from build123d import *

# Parameters (mm, degrees)
F1_DEPTH      = 1.5
F3_DEPTH      = 1.5
F4_W          = 1
F4_H          = 1
F4_W_2        = 0.5
F5_DEPTH      = 5
F5_DEPTH_BACK = 5
F6_COUNT      = 4
F6_ANGLE      = 270


with BuildPart() as f1:
    # F0 (on Top) → F1 (new body)
    with BuildSketch(Plane.XY):
        with BuildLine():
            ThreePointArc((16.8, 11), (15.1012193309, 15.1012193309), (11, 16.8))
            Line((11, 16.8), (-11, 16.8))
            ThreePointArc((-11, 16.8), (-15.1012193309, 15.1012193309), (-16.8, 11))
            Line((-16.8, 11), (-16.8, -11))
            ThreePointArc((-16.8, -11), (-15.1012193309, -15.1012193309), (-11, -16.8))
            Line((-11, -16.8), (11, -16.8))
            ThreePointArc((11, -16.8), (15.1012193309, -15.1012193309), (16.8, -11))
            Line((16.8, -11), (16.8, 11))
        make_face()
        with BuildLine():
            Line((-11, 15.3), (11, 15.3))
            ThreePointArc((11, 15.3), (14.0405591591, 14.0405591591), (15.3, 11))
            Line((15.3, 11), (15.3, -11))
            ThreePointArc((15.3, -11), (14.0405591591, -14.0405591591), (11, -15.3))
            Line((11, -15.3), (-11, -15.3))
            ThreePointArc((-11, -15.3), (-14.0405591591, -14.0405591591), (-15.3, -11))
            Line((-15.3, -11), (-15.3, 11))
            ThreePointArc((-15.3, 11), (-14.0405591591, 14.0405591591), (-11, 15.3))
        make_face(mode=Mode.SUBTRACT)
        with BuildLine():
            ThreePointArc((15.3, 11), (14.0405591591, 14.0405591591), (11, 15.3))
            Line((11, 15.3), (-11, 15.3))
            ThreePointArc((-11, 15.3), (-14.0405591591, 14.0405591591), (-15.3, 11))
            Line((-15.3, 11), (-15.3, -11))
            ThreePointArc((-15.3, -11), (-14.0405591591, -14.0405591591), (-11, -15.3))
            Line((-11, -15.3), (11, -15.3))
            ThreePointArc((11, -15.3), (14.0405591591, -14.0405591591), (15.3, -11))
            Line((15.3, -11), (15.3, 11))
        make_face()
        with BuildLine():
            Line((-11, 15), (11, 15))
            ThreePointArc((11, 15), (13.8284271247, 13.8284271247), (15, 11))
            Line((15, 11), (15, -11))
            ThreePointArc((15, -11), (13.8284271247, -13.8284271247), (11, -15))
            Line((11, -15), (-11, -15))
            ThreePointArc((-11, -15), (-13.8284271247, -13.8284271247), (-15, -11))
            Line((-15, -11), (-15, 11))
            ThreePointArc((-15, 11), (-13.8284271247, 13.8284271247), (-11, 15))
        make_face(mode=Mode.SUBTRACT)
        with BuildLine():
            ThreePointArc((15, 11), (13.8284271247, 13.8284271247), (11, 15))
            Line((11, 15), (-11, 15))
            ThreePointArc((-11, 15), (-13.8284271247, 13.8284271247), (-15, 11))
            Line((-15, 11), (-15, -11))
            ThreePointArc((-15, -11), (-13.8284271247, -13.8284271247), (-11, -15))
            Line((-11, -15), (11, -15))
            ThreePointArc((11, -15), (13.8284271247, -13.8284271247), (15, -11))
            Line((15, -11), (15, 11))
        make_face()
    extrude(amount=F1_DEPTH)

    # F2 (on face) → F3 (join)
    with BuildSketch(Plane.XY.offset(1.5)):
        with BuildLine():
            Line((16.8, -11), (16.8, 11))
            ThreePointArc((16.8, 11), (15.1012193309, 15.1012193309), (11, 16.8))
            Line((11, 16.8), (-11, 16.8))
            ThreePointArc((-11, 16.8), (-15.1012193309, 15.1012193309), (-16.8, 11))
            Line((-16.8, 11), (-16.8, -11))
            ThreePointArc((-16.8, -11), (-15.1012193309, -15.1012193309), (-11, -16.8))
            Line((-11, -16.8), (11, -16.8))
            ThreePointArc((11, -16.8), (15.1012193309, -15.1012193309), (16.8, -11))
        make_face()
        with BuildLine():
            Line((-11, 15.3), (11, 15.3))
            ThreePointArc((11, 15.3), (14.0405591591, 14.0405591591), (15.3, 11))
            Line((15.3, 11), (15.3, -11))
            ThreePointArc((15.3, -11), (14.0405591591, -14.0405591591), (11, -15.3))
            Line((11, -15.3), (-11, -15.3))
            ThreePointArc((-11, -15.3), (-14.0405591591, -14.0405591591), (-15.3, -11))
            Line((-15.3, -11), (-15.3, 11))
            ThreePointArc((-15.3, 11), (-14.0405591591, 14.0405591591), (-11, 15.3))
        make_face(mode=Mode.SUBTRACT)
    extrude(amount=F3_DEPTH)

    # F4 (on Front) → F5 (join, two sides)
    with BuildSketch(Plane.XZ) as f5_sk:
        with BuildLine():
            Line((-16.8, 10.5), (-16.8, 4))
            Line((-16.8, 4), (-15.8, 4))
            Line((-15.8, 4), (-15.8, 10.7488969095))
            ThreePointArc((-15.8, 10.7488969095), (-15.9830967627, 10.9326941499), (-16.2336477008, 11))
            Line((-16.2336477008, 11), (-16.3, 11))
            ThreePointArc((-16.3, 11), (-16.6535533906, 10.8535533906), (-16.8, 10.5))
        make_face()
        with Locations((-16.3, 3.5)):
            Rectangle(F4_W, F4_H)
        with Locations((-15.55, 3.5)):
            Rectangle(F4_W_2, F4_H)
        with BuildLine():
            Line((-15.8, 10.7488969095), (-15.8, 4))
            Line((-15.8, 4), (-15.3, 4))
            Line((-15.3, 4), (-15.3, 7.5))
            Line((-15.3, 7.5), (-15.738672954, 10.5707106781))
            ThreePointArc((-15.738672954, 10.5707106781), (-15.7608660432, 10.6627190959), (-15.8, 10.7488969095))
        make_face()
        with BuildLine():
            Line((-15.3, 7.5), (-15.3, 4))
            Line((-15.3, 4), (-14.848307792, 4))
            ThreePointArc((-14.848307792, 4), (-14.8342154179, 4.154457802), (-14.8441767052, 4.3092369361))
            Line((-14.8441767052, 4.3092369361), (-15.3, 7.5))
        make_face()
        with BuildLine():
            Line((-15.3, 4), (-15.3, 3))
            Line((-15.3, 3), (-14.9396990078, 3.7206019844))
            ThreePointArc((-14.9396990078, 3.7206019844), (-14.8836806771, 3.8569244249), (-14.848307792, 4))
            Line((-14.848307792, 4), (-15.3, 4))
        make_face()
    extrude(amount=F5_DEPTH)
    extrude(f5_sk.sketch, amount=-F5_DEPTH_BACK)

    # F6: F1 ×4 about axis
    f6_axis = Axis((0, 0, 16.5911819786), (0, 0, 1))


with BuildPart() as f1_1:
    add(f1.part)
    for i in range(1, F6_COUNT):
        add(f1.part.rotate(f6_axis, i * F6_ANGLE / (F6_COUNT - 1)))


solid = f1_1.part
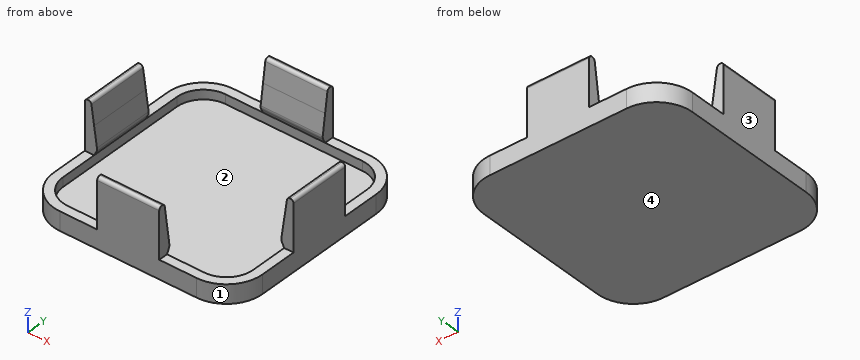
Geometry: final body of the model. Coordinates: model frame, mm. Face numbers are marked on the shaded views. Coordinates: 2 decimals unless noted, no trailing zeros. Loops run counter-clockwise (first coordinate to the right, second up) from the corner with the lowest first, then second, coordinate; pieces in that order, holes last. Notation, with made-up numbers: (54, 33.5) - (81, 33.5) arc R26 cw to (81, 52.5) - close; hole circle Ø10 at (27.25, -21). An arc over 180 degrees is marked (long way). One line per question, with ' | ' between items. Start each with the question number.
(1) Cut plane A-A on x = 6.5. Output: boundary loops of the cut face in (y, z), and give its area (3 significant figures).
(2) Ray query, L1, parallel to Y at x = -4, z = 7.5; L2, parallel to Z at x = 13.5, y = -6.5; L3, parallel to Y at x = 0.5, z = 9.5. Return the intervals inside material, ascending. Write a range as from..to.
(3) First-contact query: pin 1 (0.6 mm diameter, centred on x = 16, z = 8.5, fed in from +Y); pin 2 (1 mm diameter, centred on y = 16, z = 8, fed in from +X); pin 3 (1 mm diameter, centred on x = -16, z = 8, fed in from -Y). Flat tips, straight axial feed; report the tip coordinate or a pass-through.
(4) Cut plane B-B on z = 9.5. Output: boundary loops of the cut face in (x, y).
(5) Draft query along X for the marked faces 1, 2, 3 and 4. Return one class per face: +X half, -X half, draft (parallel to the pull), parting line (faces both ways), or undercut.
(6) Cut plane C-C on y = 2. Output: boundary loops of the cut face in (x, z).
(7) Cut plane D-D on z = 2. Output: boundary loops of the cut face in (x, y).
Here are the results:
1) outline: (-16.8, 0) - (16.8, 0) - (16.8, 3) - (15.3, 3) - (15.3, 1.5) - (-15.3, 1.5) - (-15.3, 3) - (-16.8, 3) - close | area: 54.9 mm²
2) L1: -16.8..-15.3, 15.3..16.8 | L2: 0..1.5 | L3: -16.8..-15.59, 15.59..16.8
3) pin 1: y = 5 | pin 2: x = 5 | pin 3: y = -5
4) outline: (-16.8, -5) - (-15.59, -5) - (-15.59, 5) - (-16.8, 5) - close; (-5, -16.8) - (5, -16.8) - (5, -15.59) - (-5, -15.59) - close; (-5, 15.59) - (5, 15.59) - (5, 16.8) - (-5, 16.8) - close; (15.59, -5) - (16.8, -5) - (16.8, 5) - (15.59, 5) - close
5) face 1: +X half | face 2: undercut | face 3: -X half | face 4: draft
6) outline: (-16.8, 0) - (16.8, 0) - (16.8, 10.5) arc R0.5 ccw to (16.3, 11) - (16.23, 11) arc R0.5 ccw to (15.74, 10.57) - (14.84, 4.31) arc R1 ccw to (14.94, 3.72) - (15.3, 3) - (15.3, 1.5) - (-15.3, 1.5) - (-15.3, 3) - (-14.94, 3.72) arc R1 ccw to (-14.84, 4.31) - (-15.74, 10.57) arc R0.5 ccw to (-16.23, 11) - (-16.3, 11) arc R0.5 ccw to (-16.8, 10.5) - close
7) outline: (-16.8, -11) arc R5.8 ccw to (-11, -16.8) - (11, -16.8) arc R5.8 ccw to (16.8, -11) - (16.8, 11) arc R5.8 ccw to (11, 16.8) - (-11, 16.8) arc R5.8 ccw to (-16.8, 11) - close; hole (-15.3, -11) arc R4.3 ccw to (-11, -15.3) - (11, -15.3) arc R4.3 ccw to (15.3, -11) - (15.3, 11) arc R4.3 ccw to (11, 15.3) - (-11, 15.3) arc R4.3 ccw to (-15.3, 11) - close
